Read the model definition and answer for the solid it produces. Units are mm, in the model's axes. Face numbers are marked on the shaded views. A direction names the side the tool comes from. Coordinates: 2 decimals unless noted, no trailing zeros. Loops run counter-clockwise (first coordinate to the right, second up) from the corner with the lowest first, then second, coordinate; pieces in that order, holes last.
from build123d import *

# Parameters (mm, degrees)
F1_DEPTH = 63.5
F0_W     = 25.4
F0_H     = 19.05
F2_DEPTH = 50.8
F3_DEPTH = 15.875
F5_R     = 6.35


with BuildPart() as f1:
    # F0 (on Front) → F1 (new body, symmetric)
    with BuildSketch(Plane.XZ):
        Polygon((-41.275, -9.525), (41.275, -9.525), (41.275, 9.525), (22.225, 9.525), (-41.275, 9.525), align=None)
    extrude(amount=F1_DEPTH, both=True)

    # F0 (on Front) → F2 (join)
    with BuildSketch(Plane.XZ):
        with BuildLine():
            Line((22.225, 9.525), (41.275, 9.525))
            Line((41.275, 9.525), (41.275, 27.0002))
            ThreePointArc((41.275, 27.0002), (45.92468, 38.22552), (57.15, 42.8752))
            Line((57.15, 42.8752), (60.325, 42.8752))
            Line((60.325, 42.8752), (60.325, 61.9252))
            Line((60.325, 61.9252), (57.15, 61.9252))
            ThreePointArc((57.15, 61.9252), (32.454296, 51.695904), (22.225, 27.0002))
            Line((22.225, 27.0002), (22.225, 9.525))
        make_face()
        with Locations((73.025, 52.4002)):
            Rectangle(F0_W, F0_H)
    extrude(amount=F2_DEPTH)

    # F0 (on Front) → F3 (join)
    with BuildSketch(Plane.XZ):
        with BuildLine():
            add(Edge.make_bspline(
                [(-41.275, 9.525), (-30.858979, 18.073546), (0, 64.438261), (57.15, 61.9252)],
                knots=[0, 0, 0, 0, 111.504536, 111.504536, 111.504536, 111.504536], degree=3))
            Line((-41.275, 9.525), (22.225, 9.525))
            Line((22.225, 9.525), (22.225, 27.0002))
            ThreePointArc((22.225, 27.0002), (32.454296, 51.695904), (57.15, 61.9252))
        make_face()
    extrude(amount=F3_DEPTH)

    # F0 (on Front) → F4 (revolve)
    with BuildSketch(Plane.XZ):
        Polygon((85.725, 66.675), (85.725, 61.9252), (85.725, 42.8752), (85.725, 38.1), (111.125, 38.1), (111.125, 66.675), align=None)
    revolve(axis=Axis((85.725, 0, 52.3875), (0, 0, -1)))

    # F5
    f5_edges = [f1.edges().sort_by_distance(p)[0] for p in [
        (-41.275, -63.5, 0),
        (41.275, -63.5, 0),
        (-41.275, 63.5, 0),
        (41.275, 63.5, 0),
    ]]
    fillet(f5_edges, radius=F5_R)


solid = f1.part
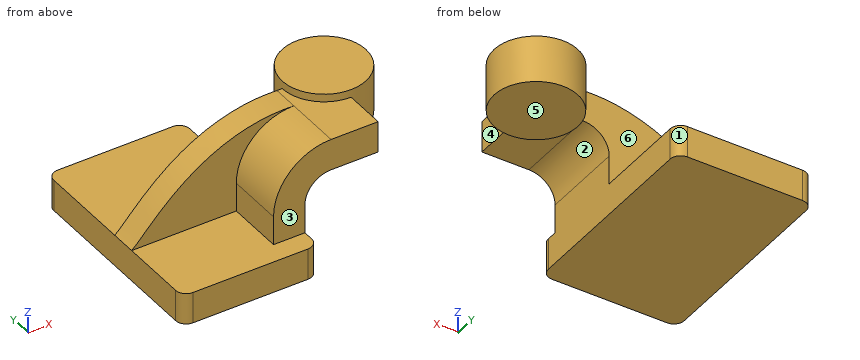
Item 1: A cutting plane is placed at A-A on y = -42. Determine the outline of the cut face in (x, z) (3 decimals), then the cut area to 3 significant figures.
Numbers:
outline: (-41.275, -9.525) - (41.275, -9.525) - (41.275, 27) arc R15.875 cw to (57.15, 42.875) - (85.725, 42.875) - (85.725, 61.925) - (57.15, 61.925) arc R34.925 ccw to (22.225, 27) - (22.225, 9.525) - (-41.275, 9.525) - close
area: 3,210 mm2
Item 2: A cutting plane is placed at D-D on y = 44. Determine the outline of the cut face in (x, z) (3 decimals).
Numbers:
outline: (-41.275, -9.525) - (41.275, -9.525) - (41.275, 9.525) - (-41.275, 9.525) - close
Item 3: A cutting plane is placed at B-B on z = -4. Determine the outline of the cut face in (x, y) (3 decimals), then the cut area to 3 significant figures.
Numbers:
outline: (-41.275, -57.15) arc R6.35 ccw to (-34.925, -63.5) - (34.925, -63.5) arc R6.35 ccw to (41.275, -57.15) - (41.275, 57.15) arc R6.35 ccw to (34.925, 63.5) - (-34.925, 63.5) arc R6.35 ccw to (-41.275, 57.15) - close
area: 10,400 mm2
Item 4: A cutting plane is placed at C-C on y = -20. Determine the outline of the cut face in (x, z) (3 decimals), then the cut area to 3 significant figures.
Numbers:
outline: (-41.275, -9.525) - (41.275, -9.525) - (41.275, 27) arc R15.875 cw to (57.15, 42.875) - (70.067, 42.875) - (70.067, 38.1) - (101.383, 38.1) - (101.383, 66.675) - (70.067, 66.675) - (70.067, 61.925) - (57.15, 61.925) arc R34.925 ccw to (22.225, 27) - (22.225, 9.525) - (-41.275, 9.525) - close
area: 3,810 mm2
Item 5: Which of the six approach directions +Z, -Z, +X, -X, +Y, -Y give full straight-line access (tool end or side, diameter ignored) to the marked faces 4, 5 and 6?
Numbers:
face 4: +Z, -Z, +X, -Y
face 5: -Z, +X, +Y, -Y
face 6: +Z, -X, +Y
Item 6: Given pin 1 (5 mm diameter, centred on y = -42, z = 16, fed in from -X) (3 decimals); pin 2 (21 mm diameter, centred on y = -36, z = 49, fed in from +X) (3 decimals); pin 3 (8.5 mm diameter, centred on x = 71.5, y = -16, fed in from -Z), each flat-ended and moving along its own axis, determine where each tip first touches the part or whether it passes through.
Numbers:
pin 1: stops at x = 22.225
pin 2: stops at x = 85.725
pin 3: stops at z = 38.1
Item 7: Find the intervals of material crossed by line 1 along X through (y, z) = (-44, 24) (3 decimals); line 2 along Z through (x, y) = (2, 55.5) (3 decimals); line 3 along X through (y, z) = (-26, 41), in increasing order.
Numbers:
line 1: x = 22.225 to 41.275
line 2: z = -9.525 to 9.525
line 3: x = 25.15 to 49.67
Item 8: Determine the mould class of the marked faces 1, 2 and 3 for opening direction X: released by +X, released by -X, zero draft, split by the parting line, or undercut.
Numbers:
face 1: released by +X
face 2: undercut
face 3: zero draft
